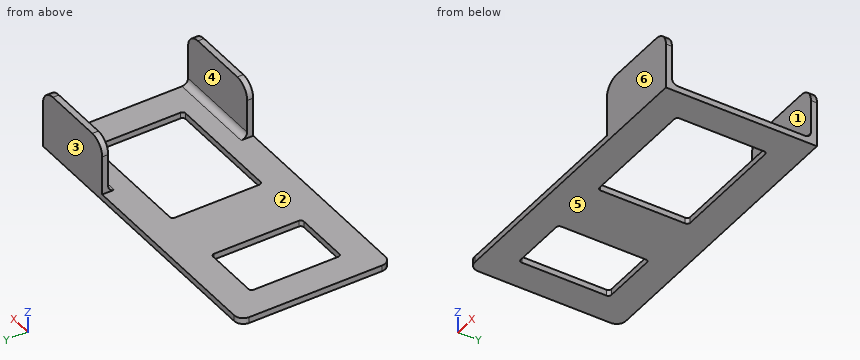
```python
from build123d import *

# Parameters (mm, degrees)
BOX001_W     = 30
BOX001_H     = 2
BOX001_DEPTH = 20
BOX002_W     = 30
BOX002_H     = 2
BOX002_DEPTH = 20
BOX_W        = 100
BOX_H        = 50
BOX_DEPTH    = 2
SKETCH_W     = 20
SKETCH_H     = 30
SKETCH_W_2   = 40
POCKET_DEPTH = 2.001
FILLET_1_R   = 3
FILLET_2_R   = 1
FILLET001_R  = 5
FILLET002_R  = 2


with BuildPart() as obj1:
    # Box001 → Box001 (new body)
    with BuildSketch(Plane(origin=(70, 0, 0), x_dir=(1, 0, 0), z_dir=(0, 0, 1))):
        with Locations((15, 1)):
            Rectangle(BOX001_W, BOX001_H)
    extrude(amount=BOX001_DEPTH)


with BuildPart() as obj2:
    # Box002 → Box002 (new body)
    with BuildSketch(Plane(origin=(70, 48, 0), x_dir=(1, 0, 0), z_dir=(0, 0, 1))):
        with Locations((15, 1)):
            Rectangle(BOX002_W, BOX002_H)
    extrude(amount=BOX002_DEPTH)


with BuildPart() as obj3:
    # Box → Box (new body)
    with BuildSketch(Plane.XY):
        with Locations((50, 25)):
            Rectangle(BOX_W, BOX_H)
    extrude(amount=BOX_DEPTH)

    # Fusion: union obj1, obj2
    add(obj1.part)
    add(obj2.part)

    # Sketch → Pocket (cut, through all)
    with BuildSketch(Plane.XY.offset(2)):
        with Locations((20, 25)):
            Rectangle(SKETCH_W, SKETCH_H)
        with Locations((70, 25)):
            Rectangle(SKETCH_W_2, SKETCH_H)
    extrude(amount=-POCKET_DEPTH, mode=Mode.SUBTRACT)

    # Fillet 1
    fillet_1_edges = [obj3.edges().sort_by_distance(p)[0] for p in [
        (0, 50, 1),
        (0, 0, 1),
    ]]
    fillet(fillet_1_edges, radius=FILLET_1_R)

    # Fillet 2
    fillet_2_edges = [obj3.edges().sort_by_distance(p)[0] for p in [
        (90, 10, 1),
        (50, 10, 1),
        (90, 40, 1),
        (50, 40, 1),
        (10, 40, 1),
        (30, 40, 1),
        (10, 10, 1),
        (30, 10, 1),
    ]]
    fillet(fillet_2_edges, radius=FILLET_2_R)

    # Fillet001
    fillet001_edges = [obj3.edges().sort_by_distance(p)[0] for p in [
        (100, 1, 20),
        (100, 49, 20),
        (70, 49, 20),
        (70, 1, 20),
    ]]
    fillet(fillet001_edges, radius=FILLET001_R)

    # Fillet002
    fillet002_edges = [obj3.edges().sort_by_distance(p)[0] for p in [
        (85, 48, 2),
        (85, 2, 2),
    ]]
    fillet(fillet002_edges, radius=FILLET002_R)


solid = obj3.part
```
Work out the finished part from the listing and answer in its coordinate system (mm). Face numbers are marked on the shaded views. A direction names the side the tool comes from. Give positions to 0.01 mm unless a question says otherwise; leave off trailing zeros. Loops run counter-clockwise (first coordinate to the right, second up) from the corner with the lowest first, then second, coordinate; pieces in that order, holes last. Notation, with made-up numbers: (34.25, 16.5) -> (82.25, 16.5) arc R17 ccw to (82.25, 20.5) -> close; hole circle Ø9 at (-8, 68.5). An arc over 180 degrees is marked (long way). Put each result on its own line as item: value. Start each with the question number.
Item 1: The mould has two halves that part along Y. Classify the marked faces 4, 5 and 6: released by +Y, released by -Y, zero draft, split by the parting line, or undercut.
Item 2: The part is cut by section A-A (x = 27). Give the vertices of the cut face in (y, z), then the cut area to 3 significant figures.
Item 3: Each of these flat-tipped pins is pushed along its axis until it touches: P1, Ø25, axis at x = 51, y = 24.5, coming from the +Z side; P2, Ø10, axis at x = 51, z = 8, coming from the +Y side; P3, Ø1.2, axis at y = 2, z = 8, coming from the -X side. Where does it stop, or does it pass through?
Item 4: Which of the six approach directions +Z, -Z, +X, -X, +Y, -Y give full straight-line access (tool end or side, diameter ignored) to the marked faces 1, 2 and 3?
Item 5: The part is cut by section D-D (x = 94). Give the vertices of the cut face in (y, z), then the cut area to 3 significant figures.
Item 6: Find the intervals of material crossed by L1, parallel to X at y = 19, z = 1.75; L2, parallel to Z at x = 44, y = 16, in increasing order. Write a range as [from, to].
Item 7: The part is cut by section C-C (y = 22). Give the vertices of the cut face in (x, z).
Item 8: The part is cut by section B-B (z = 18). Give the vertices of the cut face in (x, y).
Answers below:
1. face 4: undercut
1. face 5: zero draft
1. face 6: released by -Y
2. outline: (0, 0) -> (10, 0) -> (10, 2) -> (0, 2) -> close; (40, 0) -> (50, 0) -> (50, 2) -> (40, 2) -> close
2. area: 40.0 mm2
3. P1: z = 2
3. P2: through
3. P3: x = 70
4. face 1: +Z, +X, -X
4. face 2: +Z, -X
4. face 3: +Z, -Z, +X, -X, +Y
5. outline: (0, 0) -> (50, 0) -> (50, 20) -> (48, 20) -> (48, 4) arc R2 cw to (46, 2) -> (4, 2) arc R2 cw to (2, 4) -> (2, 20) -> (0, 20) -> close
5. area: 174 mm2
6. L1: [0, 10], [30, 50], [90, 100]
6. L2: [0, 2]
7. outline: (0, 0) -> (10, 0) -> (10, 2) -> (0, 2) -> close; (30, 0) -> (50, 0) -> (50, 2) -> (30, 2) -> close; (90, 0) -> (100, 0) -> (100, 2) -> (90, 2) -> close
8. outline: (71, 0) -> (99, 0) -> (99, 2) -> (71, 2) -> close; (71, 48) -> (99, 48) -> (99, 50) -> (71, 50) -> close
